Could you check a few things on this model? Use its own coordinates, in mm. A direction names the side the tool comes from. Give positions to 0.01 mm unless a question says otherwise; leave off trailing zeros. Write each loop counter-clockwise with the first axis right and the second up, starting at its lowest first coordinate (ties: lowest second). Pieces come first, ordered by that corner, then holes. Notation, with made-up numbers: (69.25, 62.25) - (85.25, 62.25) arc R6 cw to (85.25, 67.25) - close; hole circle Ø8 at (46.5, -27.75). An arc over 180 degrees is marked (long way). Answer in a Markdown table with one row per item.
from build123d import *

# Parameters (mm, degrees)
CROQUIS1_W              = 64.5
CROQUIS1_H              = 180
SALIENTE_EXTRUIR1_DEPTH = 30
CROQUIS2_W              = 55.309973817
CROQUIS2_H              = 20
CORTAR_EXTRUIR1_DEPTH   = 155
CORTAR_EXTRUIR2_DEPTH   = 155
CORTAR_EXTRUIR4_DEPTH   = 155
CROQUIS12_R             = 1.6
CORTAR_EXTRUIR8_DEPTH   = 10
SALIENTE_EXTRUIR2_DEPTH = 10
CROQUIS9_W              = 64.5
CROQUIS9_H              = 45.2
CORTAR_EXTRUIR10_DEPTH  = 5
CROQUIS15_R             = 1.6
CORTAR_EXTRUIR11_DEPTH  = 10
CORTAR_EXTRUIR12_REACH  = 182
CROQUIS18_W             = 21
CROQUIS18_H             = 4.5


with BuildPart() as part:
    # Croquis1 → Saliente-Extruir1 (new body)
    with BuildSketch(Plane.XY):
        Rectangle(CROQUIS1_W, CROQUIS1_H)
    extrude(amount=SALIENTE_EXTRUIR1_DEPTH)

    # Croquis2 → Cortar-Extruir1 (cut)
    with BuildSketch(Plane.XZ.offset(90)):
        with Locations((-0.404986909, 15)):
            Rectangle(CROQUIS2_W, CROQUIS2_H)
    extrude(amount=-CORTAR_EXTRUIR1_DEPTH, mode=Mode.SUBTRACT)

    # Croquis3 → Cortar-Extruir2 (cut)
    with BuildSketch(Plane(origin=(0, 0, 0), x_dir=(-1, 0, 0), z_dir=(0, 0, -1))):
        with BuildLine():
            Line((-27.25, 90), (-32.25, 90))
            Line((-32.25, 90), (-32.25, 85))
            ThreePointArc((-32.25, 85), (-30.785533906, 88.535533906), (-27.25, 90))
        make_face()
    extrude(amount=-CORTAR_EXTRUIR2_DEPTH, mode=Mode.SUBTRACT)

    # Croquis3_4 → Cortar-Extruir4 (cut)
    with BuildSketch(Plane(origin=(0, 0, 0), x_dir=(-1, 0, 0), z_dir=(0, 0, -1))):
        with BuildLine():
            Line((32.25, 90), (27.25, 90))
            ThreePointArc((27.25, 90), (30.785533906, 88.535533906), (32.25, 85))
            Line((32.25, 85), (32.25, 90))
        make_face()
    extrude(amount=-CORTAR_EXTRUIR4_DEPTH, mode=Mode.SUBTRACT)

    # Croquis12 → Cortar-Extruir8 (cut)
    with BuildSketch(Plane(origin=(0, -90, 0), x_dir=(-1, 0, 0), z_dir=(0, -1, 0))):
        with Locations((30.183391147, -15)):
            Circle(CROQUIS12_R)
        with Locations((-30.15, -15)):
            Circle(CROQUIS12_R)
    extrude(amount=-CORTAR_EXTRUIR8_DEPTH, mode=Mode.SUBTRACT)

    # Croquis14 → Saliente-Extruir2 (add)
    with BuildSketch(Plane(origin=(0, 0, 0), x_dir=(-1, 0, 0), z_dir=(0, 0, -1))):
        with BuildLine():
            ThreePointArc((-30.810899687, 83.538949092), (-25.782194726, 75.745600208), (-27.223730255, 84.90781259))
            ThreePointArc((-27.223730255, 84.90781259), (-27.750555098, 84.433527237), (-27.276269745, 83.906702394))
            ThreePointArc((-27.276269745, 83.906702394), (-26.139605296, 76.682210963), (-30.104786891, 82.827340533))
            ThreePointArc((-30.104786891, 82.827340533), (-30.102039009, 83.53620121), (-30.810899687, 83.538949092))
        make_face()
        with BuildLine():
            ThreePointArc((30.810899687, 83.538949092), (25.782194726, 75.745600208), (27.223730255, 84.90781259))
            ThreePointArc((27.223730255, 84.90781259), (27.750555098, 84.433527237), (27.276269745, 83.906702394))
            ThreePointArc((27.276269745, 83.906702394), (26.139605296, 76.682210963), (30.104786891, 82.827340533))
            ThreePointArc((30.104786891, 82.827340533), (30.102039009, 83.53620121), (30.810899687, 83.538949092))
        make_face()
        with BuildLine():
            ThreePointArc((30.810899687, -83.538949092), (25.782194726, -75.745600208), (27.223730255, -84.90781259))
            ThreePointArc((27.223730255, -84.90781259), (27.750555098, -84.433527237), (27.276269745, -83.906702394))
            ThreePointArc((27.276269745, -83.906702394), (26.139605296, -76.682210963), (30.104786891, -82.827340533))
            ThreePointArc((30.104786891, -82.827340533), (30.102039009, -83.53620121), (30.810899687, -83.538949092))
        make_face()
        with BuildLine():
            ThreePointArc((-30.810899687, -83.538949092), (-25.782194726, -75.745600208), (-27.223730255, -84.90781259))
            ThreePointArc((-27.223730255, -84.90781259), (-27.750555098, -84.433527237), (-27.276269745, -83.906702394))
            ThreePointArc((-27.276269745, -83.906702394), (-26.139605296, -76.682210963), (-30.104786891, -82.827340533))
            ThreePointArc((-30.104786891, -82.827340533), (-30.102039009, -83.53620121), (-30.810899687, -83.538949092))
        make_face()
    extrude(amount=SALIENTE_EXTRUIR2_DEPTH)

    # Croquis9 → Cortar-Extruir10 (cut)
    with BuildSketch(Plane.XY.offset(30)):
        with Locations((0, -62.4)):
            Rectangle(CROQUIS9_W, CROQUIS9_H)
    extrude(amount=-CORTAR_EXTRUIR10_DEPTH, mode=Mode.SUBTRACT)

    # Croquis15 → Cortar-Extruir11 (cut)
    with BuildSketch(Plane.XY.offset(25)):
        with Locations((30.088495575, -61.4)):
            Circle(CROQUIS15_R)
        with Locations((-30.299948917, -61.4)):
            Circle(CROQUIS15_R)
    extrude(amount=-CORTAR_EXTRUIR11_DEPTH, mode=Mode.SUBTRACT)

    # Croquis18 → Cortar-Extruir12 (cut, up to next)
    with BuildSketch(Plane(origin=(0, 90, 0), x_dir=(1, 0, 0), z_dir=(0, 1, 0)), mode=Mode.PRIVATE) as cortar_extruir12_sk1:
        with Locations((-1.25, -20.75)):
            Rectangle(CROQUIS18_W, CROQUIS18_H)
    cortar_extruir12_tool1 = extrude(cortar_extruir12_sk1.sketch, amount=-CORTAR_EXTRUIR12_REACH, mode=Mode.PRIVATE) & part.part
    add(cortar_extruir12_tool1.solids().sort_by_distance((-1.25, 90, 20.75))[0], mode=Mode.SUBTRACT)


solid = part.part
1) Imagine slicing it at A-A (x = 19). List the corners of the cut face in (y, z) for me, then the cut area to 3 significant figures.
Check values:
| item | result |
|---|---|
| outline | (-90, 0) - (90, 0) - (90, 30) - (-39.8, 30) - (-39.8, 25) - (65, 25) - (65, 5) - (-90, 5) - close; (-90, 25) - (-85, 25) - (-85, 30) - (-90, 30) - close |
| area | 2,070 mm2 |
2) We'd pull the mould along Y, two halves only. Please class faces 1 (the face through (-25.952, 75.684, -4.93)), 2 (the face through (-28.585, -85.07, 14.93)), 3 (the face through (26.007, -76.736, -4.93)), 4 (the face through (30.82, 88.5, 14.79)): +Y half, -Y half, draft (parallel to the pull), parting line (faces both ways), or undercut.
Check values:
| item | result |
|---|---|
| face 1 | undercut |
| face 2 | draft |
| face 3 | undercut |
| face 4 | +Y half |
3) If I drill on line 1 (Z direction, x = -4, y = -13); line 2 (X direction, y = -68.5, z = 9); line 3 (Y direction, x = 28, z = -1), over which ranges is the centre line in solid material (lowest first)?
Check values:
| item | result |
|---|---|
| line 1 | z = 0 to 5, 25 to 30 |
| line 2 | x = -32.25 to -28.06, 27.25 to 32.25 |
| line 3 | y = -76.47 to -75.46, 75.46 to 76.47 |
4) Imagine slicing it at D-D (z = -2.5). List the corners of the cut face in (x, y) for me.
Check values:
| item | result |
|---|---|
| outline | (-30.81, -83.54) arc R0.5 ccw to (-30.1, -82.83) arc R3.74 cw (long way) to (-27.28, -83.91) arc R0.5 ccw to (-27.22, -84.91) arc R4.74 ccw (long way) to start; (-30.81, 83.54) arc R4.74 ccw (long way) to (-27.22, 84.91) arc R0.5 ccw to (-27.28, 83.91) arc R3.74 cw (long way) to (-30.1, 82.83) arc R0.5 ccw to start; (27.22, -84.91) arc R0.5 ccw to (27.28, -83.91) arc R3.74 cw (long way) to (30.1, -82.83) arc R0.5 ccw to (30.81, -83.54) arc R4.74 ccw (long way) to start; (27.22, 84.91) arc R4.74 ccw (long way) to (30.81, 83.54) arc R0.5 ccw to (30.1, 82.83) arc R3.74 cw (long way) to (27.28, 83.91) arc R0.5 ccw to start |
5) Imagine slicing it at C-C (y = -61.4). List the corners of the cut face in (x, z) for me.
Check values:
| item | result |
|---|---|
| outline | (-32.25, 0) - (32.25, 0) - (32.25, 25) - (31.69, 25) - (31.69, 15) - (28.49, 15) - (28.49, 25) - (27.25, 25) - (27.25, 5) - (-28.06, 5) - (-28.06, 25) - (-28.7, 25) - (-28.7, 15) - (-31.9, 15) - (-31.9, 25) - (-32.25, 25) - close |
6) On a 3-axis mill with a long thin cutter (end or side, diameter ignored), from which of +Z, -Z, +X, -X, +Y, -Y can I reach the whole of each face in a straight line? I mean faces 5 (the face through (-25.952, -75.684, -4.93)), 6 (the face through (0, -85, 28)), 7 (the face through (30, -61, 15)). Say none if no direction works.
Check values:
| item | result |
|---|---|
| face 5 | -Z |
| face 6 | +Z, +X, -X |
| face 7 | +Z |
7) Will these pins go through, and if not, where does the flat tip stop? P1, Ø12, axis at x = -27.47, y = -80.17, coming from the +Z side; P2, Ø17, axis at x = 2, y = 80.5, coming from the -Z side; P3, Ø1.6, axis at x = 30.5, z = 15, coming from the -Y side; P4, Ø1.5, axis at x = 29.5, y = -66.5, coming from the +Z side.
Check values:
| item | result |
|---|---|
| P1 | stops at z = 30 |
| P2 | stops at z = 0 |
| P3 | stops at y = -80 |
| P4 | stops at z = 25 |
8) Imagine slicing it at B-B (y = 36). List the corners of the cut face in (x, z) for me.
Check values:
| item | result |
|---|---|
| outline | (-32.25, 0) - (32.25, 0) - (32.25, 30) - (-32.25, 30) - close; hole (-28.06, 5) - (27.25, 5) - (27.25, 25) - (-28.06, 25) - close |
